```python
from build123d import *

# Parameters (mm, degrees)
PAD_DEPTH = 10


with BuildPart() as part:
    # Sketch → Pad (new body)
    with BuildSketch(Plane.XY):
        with BuildLine():
            ThreePointArc((-14, 25), (-21.778175, 21.778175), (-25, 14))
            Line((-25, -14), (-25, 14))
            ThreePointArc((-25, -14), (-21.778175, -21.778175), (-14, -25))
            Line((14, -25), (-14, -25))
            ThreePointArc((14, -25), (21.778175, -21.778175), (25, -14))
            Line((25, 14), (25, -14))
            ThreePointArc((25, 14), (21.778175, 21.778175), (14, 25))
            Line((-14, 25), (14, 25))
        make_face()
        with BuildLine():
            ThreePointArc((-14, 20), (-18.242641, 18.242641), (-20, 14))
            Line((-20, -14), (-20, 14))
            ThreePointArc((-20, -14), (-18.242641, -18.242641), (-14, -20))
            Line((14, -20), (-14, -20))
            ThreePointArc((14, -20), (18.242641, -18.242641), (20, -14))
            Line((20, 14), (20, -14))
            ThreePointArc((20, 14), (18.242641, 18.242641), (14, 20))
            Line((-14, 20), (14, 20))
        make_face(mode=Mode.SUBTRACT)
    extrude(amount=PAD_DEPTH)


solid = part.part
```
Verification items for the finished model (mm, model axes). A direction names the side the tool comes from. Coordinates: 2 decimals unless noted, no trailing zeros. Write each loop counter-clockwise with the first axis right and the second up, starting at its lowest first coordinate (ties: lowest second). Pieces come first, ordered by that corner, then holes. Notation, with made-up numbers: M 67.5,81 L 82.5,81 A34 ccw 82.5,120 Z; hole C 50.25,11 d9. An arc over 180 degrees is marked long. Answer as a JSON object with one key per item and string values. Group by question number.
(1) Material ranges on line 1 (X direction, y = 6, z = 1); line 2 (Y direction, x = 19, z = 7), recorded low to high.
(2) Gauge pin test, flat ends, axial feed: pin 1 (5 mm diameter, centred on y = -17.5, z = 5.5, fed in from +X); pin 2 (2 mm diameter, centred on x = -19.5, z = 5.5, fed in from -Y); pin 3 (2 mm diameter, centred on y = -19, z = 7, fed in from -X). Record the tip position at first contact, or that the pin passes through.
(3) Release check for a two-part mould opening along X. For faces 1 (the face through (25, 0, 5)), 2 (the face through (-18.196, 18.289, 4.93)), 3 (the face through (0, 25, 5)), 4 (the face through (-25, 0, 5)) record: +X half, -X half, draft (parallel to the pull), parting line (faces both ways), or undercut.
(4) Cross-section at A-A, the plane y = 5.5. Record the cut outline in (x, z).
(5) Cross-section at C-C, the plane z = 1.75. Record the cut outline in (x, y).
(6) Tool access check on faces 5 (the face through (-18.289, -18.196, 4.93)), 6 (the face through (20.3, -1.7, 0)). Record the directions out of +Z, -Z, +X, -X, +Y, -Y that give a thin tool (end or side, any length) a straight path to the whole face; none if there is none.
Reply:
{
 "1": {"line 1": "-25 to -20, 20 to 25", "line 2": "-23.8 to -17.32, 17.32 to 23.8"},
 "2": {"pin 1": "x = 24.95", "pin 2": "y = -24.04", "pin 3": "x = -24.25"},
 "3": {"face 1": "+X half", "face 2": "undercut", "face 3": "draft", "face 4": "-X half"},
 "4": {"outline": "M -25,0 L -20,0 L -20,10 L -25,10 Z; M 20,0 L 25,0 L 25,10 L 20,10 Z"},
 "5": {"outline": "M -25,-14 A11 ccw -14,-25 L 14,-25 A11 ccw 25,-14 L 25,14 A11 ccw 14,25 L -14,25 A11 ccw -25,14 Z; hole M -20,-14 A6 ccw -14,-20 L 14,-20 A6 ccw 20,-14 L 20,14 A6 ccw 14,20 L -14,20 A6 ccw -20,14 Z"},
 "6": {"face 5": "+Z, -Z", "face 6": "-Z, +X, -X, +Y, -Y"}
}
